Job drawing, mm, ordinate dimensions from the low corner. One solid piece. A direction names the side the tool comes from. Round coordinates to 2 decimals unless told otherwise and drop trailing zeros. Write each loop counter-clockwise with the first axis right and the second up, starting at its lowest first coordinate (ties: lowest second). Pieces come first, ordered by that corner, then holes. Notation, with made-up numbers: M -27.5,24 L -11.5,24 A6 ccw -11.5,32 Z; hole C 52.25,21.5 d7. An arc over 180 degrees is marked long. Answer as a JSON object with one key per item and string values. Group by question number.
1. Band-saw the part on C-C, the plane x = 25. Count the separate pieces of the cut face and the enclosed holes in it, plus the area to 3 significant figures.
2. Band-saw the part on A-A, the plane x = 7.5. Write the cut outline in (y, z), plus the area to 3 significant figures.
3. Two-plate mould, pull along Z, no slides. Class the marked faces 5, 6, 7 and 8: +Z half, -Z half, draft (parallel to the pull), parting line (faces both ways), or undercut.
4. Drop flat-ended pins along their axis: pin 1 (1.5 mm diameter, centred on y = 25.5, z = 3.5, fed in from -X); pin 2 (2 mm diameter, centred on x = 33.5, z = 20, fed in from +Y); pin 3 (2 mm diameter, centred on x = 43.5, y = 35.5, fed in from -Z). Give the stop position or say it passes through.
5. Drill centre lines: line 1 (Y direction, x = 25, z = 42.75); line 2 (Y direction, x = 8.75, z = 37); line 3 (Z direction, x = 10, y = 32). Where is each one in solid material? Low to high. Write a range as from..to.
6. Which spindle directions (+Z, -Z, +X, -X, +Y, -Y) get a long thin tool onto all of the face, cutting with end or side? Do the marked faces 1, 2, 3 and 4. Say none if no direction does.
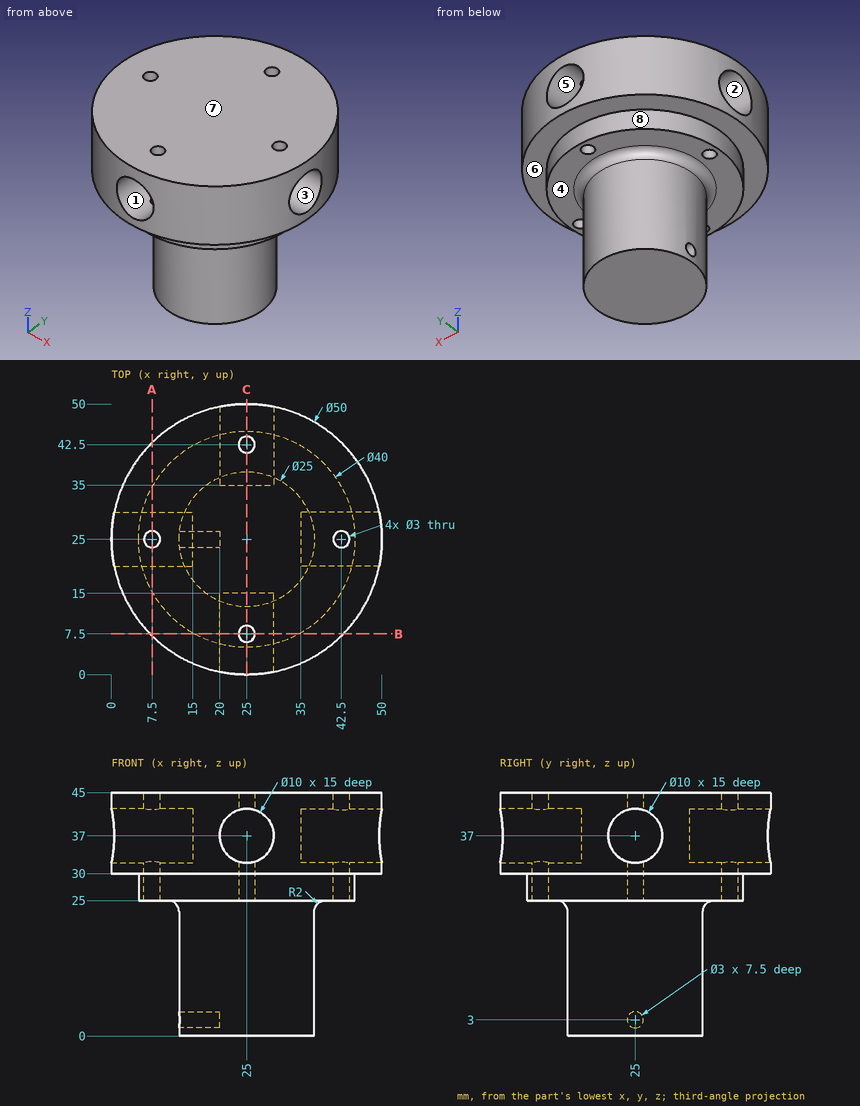
Worked answers:
{
 "1": {"separate pieces": "5", "enclosed holes": "0", "area": "1,220 mm^2"},
 "2": {"outline": "M 7.15,30 L 15.32,30 L 15.32,25 L 23.5,25 L 23.5,32.23 A5 cw 23.5,41.77 L 23.5,45 L 7.15,45 Z; M 26.5,25 L 34.68,25 L 34.68,30 L 42.85,30 L 42.85,45 L 26.5,45 L 26.5,41.77 A5 cw 26.5,32.23 Z", "area": "523 mm^2"},
 "3": {"face 5": "undercut", "face 6": "-Z half", "face 7": "+Z half", "face 8": "draft"},
 "4": {"pin 1": "stops at x = 20", "pin 2": "stops at y = 35", "pin 3": "stops at z = 30"},
 "5": {"line 1": "y = 0..6, 9..41, 44..50", "line 2": "y = 6..20, 30..44", "line 3": "z = 25..45"},
 "6": {"face 1": "-Y", "face 2": "-X", "face 3": "+X", "face 4": "-Z"}
}
